Input: part model. Units: mm. Frame: model coordinates. Face numbers are marked on the shaded views. Round coordinates to 2 decimals unless told otherwise and drop trailing zeros. Order: outer loops, then holes, each group sorted by start corner. A loop starts at its lowest first (then second) coordinate and runs counter-clockwise, first axis right, second up. Notation, with made-up numbers: (64, -30.75) -> (95, -30.75) arc R13 cw to (95, -6.75) -> close; hole circle Ø7 at (35.25, 61). An arc over 180 degrees is marked (long way). Use a Markdown table: item, result.
from build123d import *

# Parameters (mm, degrees)
SKETCH1_R           = 32.5
BOSS_EXTRUDE1_DEPTH = 436.233759
SKETCH2_R           = 22.745655965
CUT_EXTRUDE1_DEPTH  = 439.648369986
CHAMFER1_SIZE       = 3.70734


with BuildPart() as part:
    # Sketch1 → Boss-Extrude1 (new body)
    with BuildSketch(Plane(origin=(0, 0, 0), x_dir=(1, 0, 0), z_dir=(0, 1, 0))):
        with Locations(Location((0, 0, 0), (0, 0, 270))):
            Circle(SKETCH1_R)
    extrude(amount=BOSS_EXTRUDE1_DEPTH)

    # Sketch2 → Cut-Extrude1 (cut, through all)
    with BuildSketch(Plane(origin=(0, 0, 0), x_dir=(1, 0, 0), z_dir=(0, 1, 0))):
        with Locations(Location((0, 0, 0), (0, 0, 270))):
            Circle(SKETCH2_R)
    extrude(amount=CUT_EXTRUDE1_DEPTH, mode=Mode.SUBTRACT)

    # Chamfer1
    chamfer1_edges = [part.edges().sort_by_distance(p)[0] for p in [
        (0, 0, -32.5),
        (0, 436.233759, -32.5),
    ]]
    chamfer(chamfer1_edges, length=CHAMFER1_SIZE)


solid = part.part
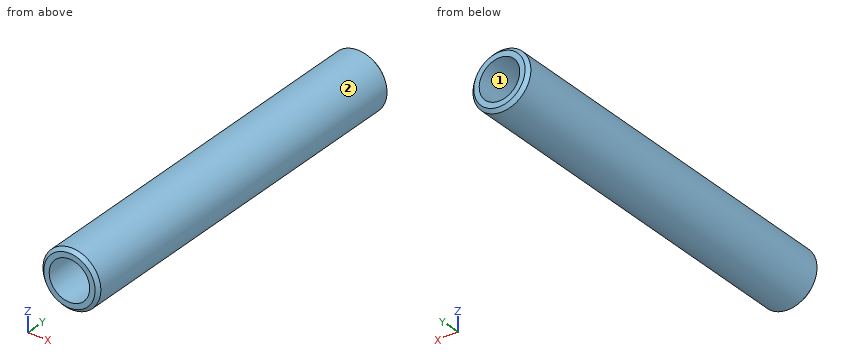
1) Cut plane A-A on z = 0. Return loops of the section in (x, y), and give its area (3 significant figures).
Results found:
| item | result |
|---|---|
| outline | (-32.5, 3.71) -> (-28.79, 0) -> (-22.75, 0) -> (-22.75, 436.23) -> (-28.79, 436.23) -> (-32.5, 432.53) -> close; (22.75, 0) -> (28.79, 0) -> (32.5, 3.71) -> (32.5, 432.53) -> (28.79, 436.23) -> (22.75, 436.23) -> close |
| area | 8,480 mm² |
2) Pin query (flat end, axial travel): pin 1 Ø1.5 at (x, y) = (20, 110.5) entering from -Z; pin 2 Ø1 at (x, y) = (-25.5, 158) entering from -Z; pin 3 Ø1 at (x, y) = (4, 129.5) entering from -Z. Return the tip coordinate at first contact, or that it passes through.
Results found:
| item | result |
|---|---|
| pin 1 | stops at z = -26.19 |
| pin 2 | stops at z = -20.77 |
| pin 3 | stops at z = -32.31 |
3) Cut plane C-C on y = 326.5. Return loops of the section in (x, z), and give its area (3 significant figures).
Results found:
| item | result |
|---|---|
| outline | circle Ø65 at (0, 0); hole circle Ø45.49 at (0, 0) |
| area | 1,690 mm² |
4) Pull-direction query (Z, two-part tool) for the marked faces 1 and 2; classes: +Z half, -Z half, draft (parallel to the pull), parting line (faces both ways), or undercut.
Results found:
| item | result |
|---|---|
| face 1 | undercut |
| face 2 | parting line |
5) Line query: L1, parallel to X at y = 147, z = 0; L2, parallel to Z at x = -0.5, y = 249; L3, parallel to Z at x = -18, y = 81. Output: solid intervals per line, ascending. Write a range as [from, to].
Results found:
| item | result |
|---|---|
| L1 | x = [-32.5, -22.75], [22.75, 32.5] |
| L2 | z = [-32.5, -22.74], [22.74, 32.5] |
| L3 | z = [-27.06, -13.91], [13.91, 27.06] |
6) Cut plane B-B on x = 0. Return loops of the section in (y, z).
Results found:
| item | result |
|---|---|
| outline | (0, -28.79) -> (3.71, -32.5) -> (432.53, -32.5) -> (436.23, -28.79) -> (436.23, -22.75) -> (0, -22.75) -> close; (0, 22.75) -> (436.23, 22.75) -> (436.23, 28.79) -> (432.53, 32.5) -> (3.71, 32.5) -> (0, 28.79) -> close |
